Build history of the part. All positions in model axes, mm. Round coordinates to 2 decimals unless told otherwise and drop trailing zeros. Loops run counter-clockwise (first coordinate to the right, second up) from the corner with the lowest first, then second, coordinate; pieces in that order, holes last.
from build123d import *

# Parameters (mm, degrees)
F0_R          = 13.0175
F0_R_2        = 7.9375
F1_DEPTH      = 19.05
F1_DEPTH_BACK = 19.05
F4_END_RADIUS = 13.0175
F3_R          = 8.89
F3_R_2        = 6.35
F4_REACH      = 63.563217139


with BuildPart() as f1:
    # F0 (on Top) → F1 (new body, two sides)
    with BuildSketch(Plane.XY) as f1_sk:
        with Locations((0, 2.0309128979)):
            Circle(F0_R)
        with Locations((0, 2.0309128979)):
            Circle(F0_R_2, mode=Mode.SUBTRACT)
    extrude(amount=F1_DEPTH)
    extrude(f1_sk.sketch, amount=-F1_DEPTH_BACK)

    f4_end = (Plane(origin=(0, 2.0309128979, -9.525), x_dir=(1, 0, 0), z_dir=(0, 0, 1)) * Cylinder(F4_END_RADIUS, 233.0934565066, mode=Mode.PRIVATE)).faces().sort_by_distance((-13.0175, 2.0309128979, -9.525))[0]
    # F3 (on offset) → F4 (join, up to the whole of a round face its end follows)
    with BuildSketch(Plane.YZ.offset(25.4)):
        Circle(F3_R)
        Circle(F3_R_2, mode=Mode.SUBTRACT)
    f4_long = extrude(amount=-F4_REACH, mode=Mode.PRIVATE)
    add(split(f4_long, bisect_by=f4_end, keep=Keep.ALL, mode=Mode.PRIVATE).solids().sort_by_distance((25.4, -8.6385528286, 0))[0])


solid = f1.part
(1) Probe line 1 (Y direction, x = 21, z = 0); line 2 (Y direction, x = 0, z = 4). List the from-to ranges inside material, lowest first.
Responses:
line 1: y = -8.89 to -6.35, 6.35 to 8.89
line 2: y = -10.99 to -5.91, 9.97 to 15.05
(2) Pin check, flat tips, straight feed: P1, Ø10, axis at x = 4, z = 2, coming from the +Y side; P2, Ø3, axis at x = 21.5, y = -1.5, coming from the +Z side; P3, Ø6, axis at y = -7.5, z = 11.5, coming from the +X side; P4, Ø6, axis at x = 5, z = -7.5, coming from the -Y side. Stop position of each tip, or through.
Responses:
P1: stops at y = 15.05
P2: stops at z = 8.89
P3: stops at x = 11.26
P4: stops at y = -10.83
(3) Slice it at B-B on y = 4.5. List the corners of the cut face in (x, z).
Responses:
outline: (-12.78, -19.05) - (-7.54, -19.05) - (-7.54, 19.05) - (-12.78, 19.05) - close; (7.54, -19.05) - (12.78, -19.05) - (12.78, -7.67) - (25.4, -7.67) - (25.4, -4.48) - (12.78, -4.48) - (12.78, 4.48) - (25.4, 4.48) - (25.4, 7.67) - (12.78, 7.67) - (12.78, 19.05) - (7.54, 19.05) - close
(4) Pull direction Z, two halves, no side cores. Call faces 1 (the face through (6, 8, -19.05)), 2 (the face through (19.5, -5.04, -3.86)), 3 (the face through (-1.03, 9.9, -0.27)), 4 (the face through (18.41, -8.88, 0.39)): +Z half, -Z half, draft (parallel to the pull), parting line (faces both ways), or undercut.
Responses:
face 1: -Z half
face 2: undercut
face 3: draft
face 4: parting line
(5) Slice it at D-D on x = 21.5. List the corners of the cut face in (y, z), plus the area to 3 significant figures.
Responses:
outline: circle Ø17.78 at (0, 0); hole circle Ø12.7 at (0, 0)
area: 122 mm2
(6) Slice it at A-A on x = 0. List the corners of the cut face in (y, z).
Responses:
outline: (-10.99, -19.05) - (-5.91, -19.05) - (-5.91, 19.05) - (-10.99, 19.05) - close; (9.97, -19.05) - (15.05, -19.05) - (15.05, 19.05) - (9.97, 19.05) - close
